Geometry check sheet. Reference: the model listing, model coordinates, mm. A direction names the side the tool comes from. Give positions to 0.01 mm unless a question says otherwise; leave off trailing zeros. Loops run counter-clockwise (first coordinate to the right, second up) from the corner with the lowest first, then second, coordinate; pieces in that order, holes last. Notation, with made-up numbers: (-31.75, -7) -> (27.25, -7) arc R26 ccw to (27.25, 28) -> close; hole circle Ø3 at (86, -8.5). An arc over 180 degrees is marked (long way). One line per question, with ' | ' between items.
from build123d import *

# Parameters (mm, degrees)
SKETCH1_R                       = 2.0701
BOSS_EXTRUDE1_DEPTH             = 2.286
F_5_32_0_15625_DIAMETER_HOLE1_D = 3.96875


with BuildPart() as part:
    # Sketch1 → Boss-Extrude1 (new body)
    with BuildSketch(Plane.XY.offset(2.286)):
        with BuildLine():
            Line((12.7, -54.991), (12.7, -6.35))
            ThreePointArc((12.7, -6.35), (14.559871939, -1.859871939), (19.05, 0))
            Line((19.05, 0), (42.291, 0))
            Line((42.291, 0), (44.45, 2.159))
            Line((44.45, 2.159), (44.45, 23.241))
            Line((44.45, 23.241), (42.291, 25.4))
            Line((42.291, 25.4), (-42.291, 25.4))
            Line((-42.291, 25.4), (-44.45, 23.241))
            Line((-44.45, 23.241), (-44.45, 2.159))
            Line((-44.45, 2.159), (-42.291, 0))
            Line((-42.291, 0), (-19.05, 0))
            ThreePointArc((-19.05, 0), (-14.559871939, -1.859871939), (-12.7, -6.35))
            Line((-12.7, -6.35), (-12.7, -54.991))
            Line((-12.7, -54.991), (-10.541, -57.15))
            Line((-10.541, -57.15), (10.541, -57.15))
            Line((10.541, -57.15), (12.7, -54.991))
        make_face()
        with Locations((0, -50.8)):
            Circle(SKETCH1_R, mode=Mode.SUBTRACT)
    extrude(amount=-BOSS_EXTRUDE1_DEPTH)

    # 5/32 (0.15625) Diameter Hole1 (through all)
    with Locations(Plane.XY.offset(2.286)):
        with Locations((-38.1, 12.7), (-25.4, 12.7), (-12.7, 12.7), (0, 12.7), (12.7, 12.7), (25.4, 12.7), (38.1, 12.7), (0, 0), (0, -12.7), (0, -25.4), (0, -38.1), (0, -50.8)):
            Hole(F_5_32_0_15625_DIAMETER_HOLE1_D / 2)


solid = part.part
Item 1: Sectioned sample at A-A (x = 38.1). Record the cut outline in (y, z), plus the area to 3 significant figures.
Result:
outline: (0, 0) -> (10.72, 0) -> (10.72, 2.29) -> (0, 2.29) -> close; (14.68, 0) -> (25.4, 0) -> (25.4, 2.29) -> (14.68, 2.29) -> close | area: 49.0 mm2
Item 2: Set-up check for faces 1 (the face through (-31, 0, 1)), 2 (the face through (44.45, 13, 1)): record each of +Z, -Z, +X, -X, +Y, -Y from which the full face is reachable in a straight line by a thin tool's end or side.
Result:
face 1: +Z, -Z, -X, -Y | face 2: +Z, -Z, +X, +Y, -Y
Item 3: Depth check by flat-ended pin: pin 1 Ø0.7 at (y, z) = (-19, 1) entering from -X; pin 2 Ø0.7 at (x, z) = (34.5, 1) entering from -Y; pin 3 Ø2.5 at (x, y) = (-12.7, 12.7) entering from +Z. Enter the tip coordinate at first touch or a pass-through.
Result:
pin 1: x = -12.7 | pin 2: y = 0 | pin 3: through
Item 4: Sectioned sample at C-C (y = 12.7). Give the number of separate pieces and of enclosed holes in the cut face, plus the area to 3 significant figures.
Result:
separate pieces: 8 | enclosed holes: 0 | area: 140 mm2
Item 5: Scan lines: probe 1 along Y at (x, z) = (25.4, 1.8); probe 2 along Y at (x, z) = (-11.5, 2.1); probe 3 along X at (y, z) = (-7.5, 1.7). Record each from-to range of solid material in increasing order.
Result:
probe 1: 0 to 10.72, 14.68 to 25.4 | probe 2: -56.19 to 11.12, 14.28 to 25.4 | probe 3: -12.7 to 12.7
Item 6: Release check for a two-part mould opening along X. For faces 3 (the face through (12.7, -31, 1)), 4 (the face through (0.258, -23.433, 1.127)), 5 (the face through (-43.355, 24.336, 1.159)) record: pulls with the +X half, pulls with the -X half, needs draft (parallel to the pull), parting line crosses it, or undercut.
Result:
face 3: pulls with the +X half | face 4: undercut | face 5: pulls with the -X half
Item 7: Sectioned sample at B-B (y = -25.4). Record the cut outline in (x, z), plus the area to 3 significant figures.
Result:
outline: (-12.7, 0) -> (-1.98, 0) -> (-1.98, 2.29) -> (-12.7, 2.29) -> close; (1.98, 0) -> (12.7, 0) -> (12.7, 2.29) -> (1.98, 2.29) -> close | area: 49.0 mm2
